Design review of the part built by this model. Coordinates are the model's own, in mm. A direction names the side the tool comes from. Give positions to 0.01 mm unless a question says otherwise; leave off trailing zeros. Loops run counter-clockwise (first coordinate to the right, second up) from the corner with the lowest first, then second, coordinate; pieces in that order, holes last. Notation, with made-up numbers: (70.5, 89) - (78.5, 89) arc R20 ccw to (78.5, 123) - close; hole circle Ø3 at (8.25, 22.5). An arc over 180 degrees is marked (long way). One line per item, written item: value. Start each with the question number.
```python
from build123d import *

# Parameters (mm, degrees)
CROQUIS1_R              = 3.25
SALIENTE_EXTRUIR1_DEPTH = 3


with BuildPart() as part:
    # Croquis1 → Saliente-Extruir1 (new body)
    with BuildSketch(Plane(origin=(0, 0, 0), x_dir=(1, 0, 0), z_dir=(0, 1, 0))):
        Polygon((0, 12.5), (0, 0), (10.5, 0), (10.5, 3), (25.5, 3), (25.5, 0), (40.5, 0), (40.5, 3), (55.5, 3), (55.5, 0), (70.5, 0), (70.5, 3), (85.5, 3), (85.5, 0), (100.5, 0), (100.5, 3), (115.5, 3), (115.5, 0), (130.5, 0), (130.5, 3), (145.5, 3), (145.5, 0), (153, 0), (153, 17.5), (150, 17.5), (150, 25), (150, 32.5), (153, 32.5), (153, 50), (145.5, 50), (145.5, 47), (130.5, 47), (130.5, 50), (115.5, 50), (115.5, 47), (100.5, 47), (100.5, 50), (93, 50), (85.5, 50), (85.5, 47), (70.5, 47), (70.5, 50), (67.60876348, 50), (55.5, 50), (55.5, 47), (40.5, 47), (40.5, 50), (25.5, 50), (25.5, 47), (10.5, 47), (10.5, 50), (3, 50), (0, 50), (0, 40), (0, 27.5), (3, 27.5), (3, 20), (3, 12.5), align=None)
        with Locations(Location((93, 30, 0), (0, 0, 270))):
            Circle(CROQUIS1_R, mode=Mode.SUBTRACT)
        with Locations(Location((93, 40, 0), (0, 0, 270))):
            Circle(CROQUIS1_R, mode=Mode.SUBTRACT)
    extrude(amount=SALIENTE_EXTRUIR1_DEPTH)


solid = part.part
```
(1) Draft analysis for pull direction X (two halves, no side actions). For faces 1 (the flat face through (93, 1, 0)), 2 (the flat face through (78, 1, -47)), 3 (the flat face through (153, 1, -41)), state which applies: pulls with the +X half, pulls with the -X half, needs draft (parallel to the pull), parting line crosses it, or undercut.
(2) Take a section at C-C on y = 1.8. State how many separate pieces and enclosed holes the cut face has, and give its area (3 significant figures).
(3) For pin 1 Ø0.9 at (y, z) = (2, -48) entering from -X; pin 2 Ø0.9 at (x, y) = (136.5, 1) entering from +Z; pin 3 Ø0.9 at (x, y) = (107.5, 2) entering from -Z, all flat-tipped, find the tip position at first contact; note any pin that passes through.
(4) To check wall thickness, follow L1, parallel to X at y = 1.35, z = -40; L2, parallel to X at y = 1.2, z = -30; L3, parallel to Z at x = 136, y = 2.8. State the ranges of each line that lie inside material, in increasing order. Write a range as from..to.
(5) Take a section at D-D on z = -40. State the section outline as (x, y) points, and give its area (4 significant figures).
(6) Machinability: for faces 4 (the flat face through (40.5, 1, -1)), 5 (the flat face through (18, 1, -47)), 6 (the flat face through (152, 1, -17.5)), which of the approach directions +Z, -Z, +X, -X, +Y, -Y give a long, thin tool a straight path to every point of the face, cutting with its end or side? Answer none if there is none.
(7) Take a section at B-B on z = -30. State the section outline as (x, y) points.
(8) Take a section at A-A on x = 93. State the section outline as (y, z) points, and give its area (3 significant figures).
Here are the results:
1. face 1: needs draft
1. face 2: undercut
1. face 3: pulls with the +X half
2. separate pieces: 1
2. enclosed holes: 2
2. area: 7,040 mm²
3. pin 1: x = 0
3. pin 2: z = -3
3. pin 3: z = -47
4. L1: 0..89.75, 96.25..153
4. L2: 0..89.75, 96.25..150
4. L3: -47..-3
5. outline: (0, 0) - (89.75, 0) - (89.75, 3) - (0, 3) - close; (96.25, 0) - (153, 0) - (153, 3) - (96.25, 3) - close
5. area: 439.5 mm²
6. face 4: +Z, +Y, -Y
6. face 5: -Z, +Y, -Y
6. face 6: +X, +Y, -Y
7. outline: (0, 0) - (89.75, 0) - (89.75, 3) - (0, 3) - close; (96.25, 0) - (150, 0) - (150, 3) - (96.25, 3) - close
8. outline: (0, -50) - (3, -50) - (3, -43.25) - (0, -43.25) - close; (0, -36.75) - (3, -36.75) - (3, -33.25) - (0, -33.25) - close; (0, -26.75) - (3, -26.75) - (3, 0) - (0, 0) - close
8. area: 111 mm²
